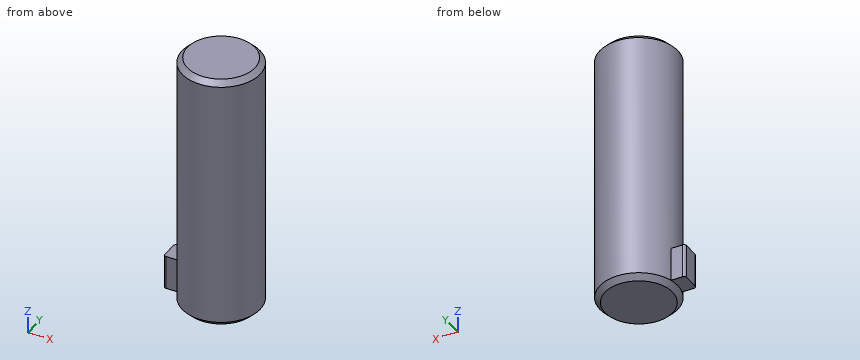
Autodesk Inventor part; units mm, degrees
ref_plane "Work Plane1" through (-10, 0, 0) normal (1, 0, 0) x (0, 1, 0)
ref_plane "XZ Plane" through (0, 0, 0) normal (0, 1, 0) x (-1, 0, 0)
ref_plane "XY Plane" through (0, 0, 0) normal (0, 0, 1) x (1, 0, 0)
sketch "Sketch1" plane through (0, 0, 0) normal (0, 0, 1) x (1, 0, 0)
  circle A0 centre (0, 0) radius 15
  dimension "d0" = 30
extrude "Extrusion1" add sketch "Sketch1" along normal blind 100
chamfer "Chamfer1" distance 2 angle 45 1 edges at (-15, 0, 100)
chamfer "Chamfer2" distance 2 angle 45 1 edges at (-15, 0, 0)
ref_plane "Work Plane1" through (-10, 0, 0) normal (1, 0, 0) x (0, 1, 0)
sketch "Sketch2" plane through (-10, 0, 0) normal (1, 0, 0) x (0, 1, 0)
  line L0 (-15, 2) -> (15, 2)
  line L1 (4, 2) -> (-4, 2)
  line L2 (-4, 2) -> (-4, 15)
  line L3 (-4, 15) -> (4, 15)
  line L4 (4, 15) -> (4, 2)
  line L5 (4, 2) -> (-4, 15) construction
  line L6 (-4, 2) -> (4, 15) construction
  line L7 (0, -20) -> (0, 120)
  line L8 (15, 98) -> (-15, 98)
  line L9 (-15, 2) -> (15, 2)
  line L10 (-15, 2) -> (-15, 98)
  line L11 (15, 2) -> (15, 98)
  point P0 (0, 0)
  point P1 (0, 8.5)
  dimension "d10" = 8
  dimension "d11" = 13
  dimension "d12" = 15
extrude "Extrusion2" add sketch "Sketch2" against normal blind 10 contours L2 L3 L7 L0 | L7 L3 L4 L0
fillet "Fillet1" radius 1 2 edges at (-20, 4, 8.5) (-20, -4, 8.5)
properties part number "Shaft" material "Lead"
Work out the finished part from the listing and answer in its coordinate system (mm). Give positions to 0.01 mm unless a question says otherwise; leave off trailing zeros. Loops run counter-clockwise (first coordinate to the right, second up) from the corner with the lowest first, then second, coordinate; pieces in that order, holes last. Notation, with made-up numbers: (65, 53.25) - (77, 53.25) arc R25 ccw to (77, 83.25) - close; hole circle Ø2 at (61, 23). An arc over 180 degrees is marked (long way). Answer in a Markdown table with one row per item. Add a question column.
Q1. The part is cut by section B-B (z = 69). Determine the outline of the cut face in (x, y), and give its area (3 significant figures).
Q2. Each of these flat-tipped pins is pushed along its axis until it touches: P1, Ø1.5, axis at x = -4.5, y = 0.5, coming from the -Z side; P2, Ø1.5, axis at y = -12, z = 23.5, coming from the +X side; P3, Ø12, axis at x = -14, z = 31, coming from the -Y side; P4, Ø4.5, axis at x = -18, y = 2, coming from the -Z side. Where does it stop, or does it pass through?
Q3. The part is cut by section A-A (y = 0). Determine the outline of the cut face in (x, z).
Q4. Consider line 1 along X through (y, z) = (-0.5, 46); line 2 along X through (y, z) = (12.25, 14.5); line 3 along Y through (x, z) = (-9.5, 72). Determine where each line is inside the solid, lowest interval first.
Solution:
| question | item | result |
|---|---|---|
| 1 | outline | circle Ø30 at (0, 0) |
| 1 | area | 707 mm² |
| 2 | P1 | stops at z = 0 |
| 2 | P2 | stops at x = 9.92 |
| 2 | P3 | stops at y = -12.69 |
| 2 | P4 | stops at z = 2 |
| 3 | outline | (-20, 2) - (-15, 2) - (-13, 0) - (13, 0) - (15, 2) - (15, 98) - (13, 100) - (-13, 100) - (-15, 98) - (-15, 15) - (-20, 15) - close |
| 4 | line 1 | x = -14.99 to 14.99 |
| 4 | line 2 | x = -8.66 to 8.66 |
| 4 | line 3 | y = -11.61 to 11.61 |
